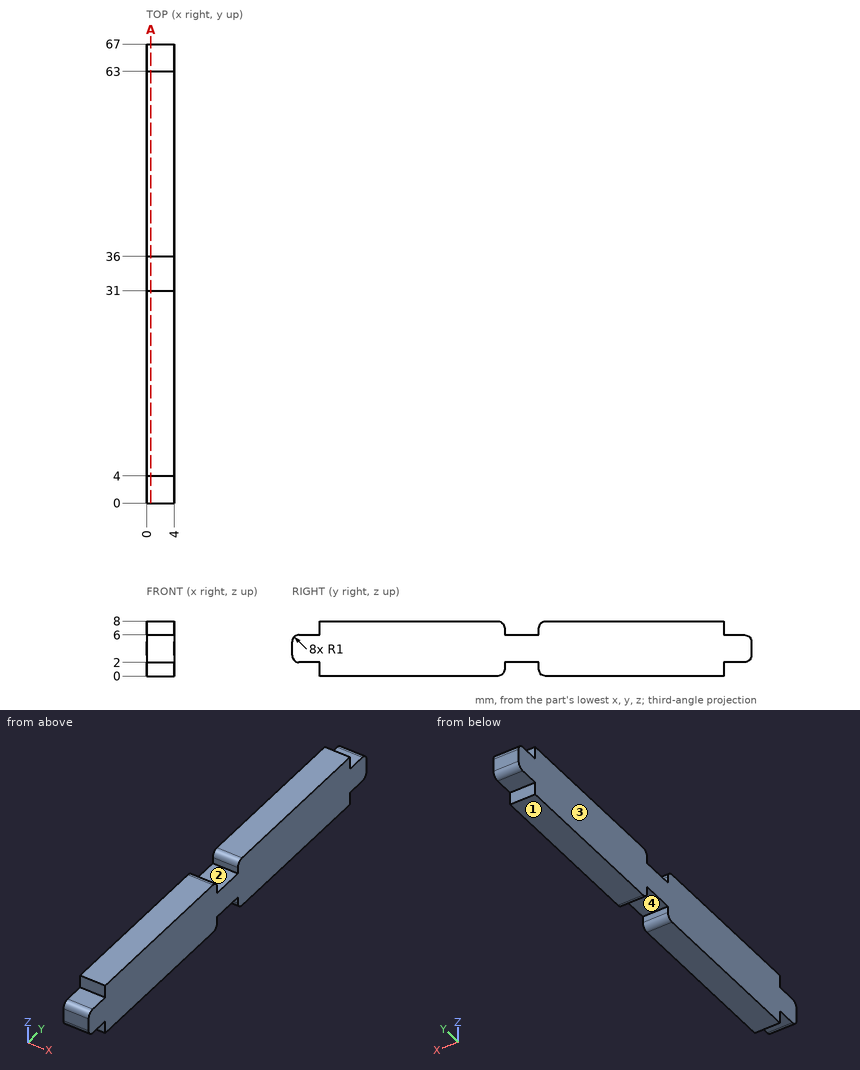
The drawing under review shows one solid part. Ordinate dimensions are in mm from its lowest x, y, z. A direction names the side the tool comes from. Give positions to 0.01 mm unless a question says otherwise; leave off trailing zeros. Order: outer loops, then holes, each group sorted by start corner. A loop starts at its lowest first (then second) coordinate and runs counter-clockwise, first axis right, second up. Notation, with made-up numbers: (-11, 4) - (14, 4) arc R27 ccw to (14, 41) - close; hole circle Ø8 at (36.25, 60.25). An arc over 180 degrees is marked (long way). Answer as a JSON object with one key per item and string values. Group by question number.
Item 1: Clearance check with flat-ended pins moving along their axes: pin 1 Ø0.9 at (x, y) = (1.5, 65) entering from -Z; pin 2 Ø1.2 at (x, y) = (1, 33.5) entering from +Z; pin 3 Ø0.6 at (x, z) = (1, 1.5) entering from +Y; pin 4 Ø1 at (x, y) = (2.5, 50) entering from -Z. State where each tip first meets the part, or that it passes through.
Item 2: Take a section at A-A on x = 0.6. Give the boundary of the cut face in (y, z), and give its area (3 significant figures).
Item 3: Draft analysis for pull direction Y (two halves, no side actions). For the marked faces 3 and 4, state which applies: pulls with the +Y half, pulls with the -Y half, needs draft (parallel to the pull), parting line crosses it, or undercut.
Item 4: Machinability: for the marked faces 1 and 2, which of the approach directions +Z, -Z, +X, -X, +Y, -Y give a long, thin tool a straight path to every point of the face, cutting with its end or side? Answer none if there is none.
Item 5: Wall thickness on line 1 along Y through (x, z) = (3.8, 6.5); line 2 along Z through (x, y) = (1.1, 3); line 3 along Z through (x, y) = (2.55, 36.5): over which ranges is each line inside the solid? List them lowest first.
Reported:
{
 "1": {"pin 1": "z = 2", "pin 2": "z = 6", "pin 3": "y = 63", "pin 4": "z = 0"},
 "2": {"outline": "(0, 3) arc R1 ccw to (1, 2) - (4, 2) - (4, 0) - (30, 0) arc R1 ccw to (31, 1) - (31, 2) - (36, 2) - (36, 1) arc R1 ccw to (37, 0) - (63, 0) - (63, 2) - (66, 2) arc R1 ccw to (67, 3) - (67, 5) arc R1 ccw to (66, 6) - (63, 6) - (63, 8) - (37, 8) arc R1 ccw to (36, 7) - (36, 6) - (31, 6) - (31, 7) arc R1 ccw to (30, 8) - (4, 8) - (4, 6) - (1, 6) arc R1 ccw to (0, 5) - close", "area": "482 mm^2"},
 "3": {"face 3": "needs draft", "face 4": "undercut"},
 "4": {"face 1": "-Z, +X, -X, +Y, -Y", "face 2": "+Z, +X, -X"},
 "5": {"line 1": "4 to 31, 36 to 63", "line 2": "2 to 6", "line 3": "0.13 to 7.87"}
}
